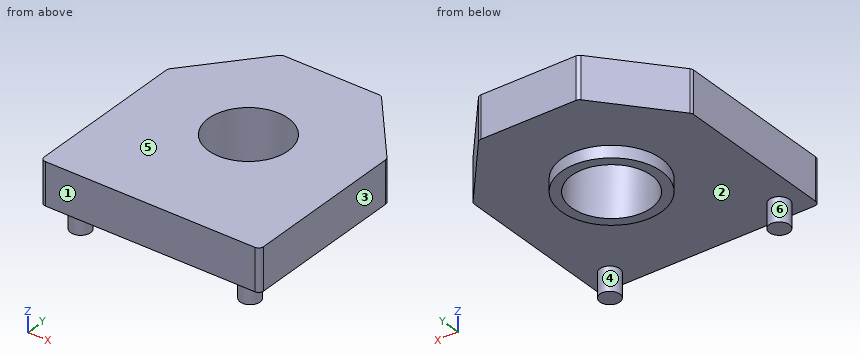
from build123d import *

# Parameters (mm, degrees)
EXTRUSION1_DEPTH = 2.11
CONG_1_R         = 0.25
ESQUISSE2_R      = 2
EXTRUSION2_DEPTH = 17.414996193
ESQUISSE3_R      = 2.5
ESQUISSE3_R_2    = 2
EXTRUSION3_DEPTH = 0.6
ESQUISSE4_R      = 0.5
EXTRUSION4_DEPTH = 1.2


with BuildPart() as part:
    # Esquisse1 → Extrusion1 (new body)
    with BuildSketch(Plane.XY):
        Polygon((0, 8.42), (3.00397668, 12), (7.99602332, 12), (11, 8.42), (11, 0), (0, 0), align=None)
    extrude(amount=EXTRUSION1_DEPTH)

    # Congé1
    cong_1_edges = [part.edges().sort_by_distance(p)[0] for p in [
        (0, 8.42, 1.055),
        (3.00397668, 12, 1.055),
        (7.99602332, 12, 1.055),
        (11, 8.42, 1.055),
        (11, 0, 1.055),
        (0, 0, 1.055),
    ]]
    fillet(cong_1_edges, radius=CONG_1_R)

    # Esquisse2 → Extrusion2 (cut, through all)
    with BuildSketch(Plane.XY.offset(2.11)):
        with Locations((5.5, 6.5)):
            Circle(ESQUISSE2_R)
    extrude(amount=-EXTRUSION2_DEPTH, mode=Mode.SUBTRACT)

    # Esquisse3 → Extrusion3 (add)
    with BuildSketch(Plane(origin=(0, 0, 0), x_dir=(-1, 0, 0), z_dir=(0, 0, -1))):
        with Locations((-5.5, 6.5)):
            Circle(ESQUISSE3_R)
        with Locations(Location((-5.5, 6.5, 0), (0, 0, 180))):
            Circle(ESQUISSE3_R_2, mode=Mode.SUBTRACT)
    extrude(amount=EXTRUSION3_DEPTH)

    # Esquisse4 → Extrusion4 (add)
    with BuildSketch(Plane(origin=(0, 0, 0), x_dir=(-1, 0, 0), z_dir=(0, 0, -1))):
        with Locations((-9.75, 1.01)):
            Circle(ESQUISSE4_R)
        with Locations((-1.25, 1.01)):
            Circle(ESQUISSE4_R)
    extrude(amount=EXTRUSION4_DEPTH)


solid = part.part
Part model, mm, in its own coordinate system. Face numbers are marked on the shaded views. A direction names the side the tool comes from. Coordinates: 2 decimals unless noted, no trailing zeros. Order: outer loops, then holes, each group sorted by start corner. A loop starts at its lowest first (then second) coordinate and runs counter-clockwise, first axis right, second up. Notation, with made-up numbers: M -24.5,-12.75 L 12.5,-12.75 A30 ccw 12.5,21.25 Z; hole C -34.75,89 d2. An arc over 180 degrees is marked long. One line per question, with ' | ' between items.
Q1. Slice it at C-C (y = 4.75). Give the cut face in (x, z), and give its area (3 significant figures).
A:
outline: M 0,0 L 3.71,0 L 3.71,-0.6 L 4.53,-0.6 L 4.53,2.11 L 0,2.11 Z; M 6.47,-0.6 L 7.29,-0.6 L 7.29,0 L 11,0 L 11,2.11 L 6.47,2.11 Z | area: 20.1 mm^2
Q2. Drill centre lines: line 1 (X direction, y = 6.5, z = 1.6); line 2 (Y direction, x = 5.5, z = 1.05); line 3 (Z direction, x = 8.5, y = 1.5). Where is each one in solid material? Low to high.
A:
line 1: x = 0 to 3.5, 7.5 to 11 | line 2: y = 0 to 4.5, 8.5 to 12 | line 3: z = 0 to 2.11
Q3. 3-axis set-ups, long thin cutter, end or side, ignore diameter. For the marked faces 1 and 2: which of +Z, -Z, +X, -X, +Y, -Y reach the whole face in a straight line?
A:
face 1: +Z, -Z, +X, -X, -Y | face 2: -Z
Q4. Slice it at A-A (x = 5.5). Give the cut face in (y, z), and give its area (3 significant figures).
A:
outline: M 0,0 L 4,0 L 4,-0.6 L 4.5,-0.6 L 4.5,2.11 L 0,2.11 Z; M 8.5,-0.6 L 9,-0.6 L 9,0 L 12,0 L 12,2.11 L 8.5,2.11 Z | area: 17.5 mm^2
Q5. Slice it at B-B (z = 1.85). Give the cut face in (x, y).
A:
outline: M 0,0.25 A0.25 ccw 0.25,0 L 10.75,0 A0.25 ccw 11,0.25 L 11,8.33 A0.25 ccw 10.94,8.49 L 8.07,11.91 A0.25 ccw 7.88,12 L 3.12,12 A0.25 ccw 2.93,11.91 L 0.06,8.49 A0.25 ccw 0,8.33 Z; hole C 5.5,6.5 d4
Q6. Two-plate mould, pull along X, no slides. Class the marked faces 3, 4, 5 and 6: +X half, -X half, draft (parallel to the pull), parting line (faces both ways), or undercut.
A:
face 3: +X half | face 4: undercut | face 5: draft | face 6: undercut
Q7. Slice it at D-D (z = -0.9). Give the cut face in (x, y), and give its area (3 significant figures).
A:
outline: C 1.25,1.01 d1; C 9.75,1.01 d1 | area: 1.57 mm^2
Q8. Pin check, flat tip, straight feed: P1, Ø5.5, axis at x = 5.5, y = 6.5, coming from the -Z side. Stop position of the tip, or through.
A:
P1: stops at z = -0.6
